```python
from build123d import *

# Parameters (mm, degrees)
SKIZZE1_W                       = 7.72
SKIZZE1_H                       = 10
SKIZZE1_W_2                     = 1.2
SKIZZE1_H_2                     = 20
SKIZZE1_W_3                     = 27.68
SKIZZE1_H_3                     = 5
AUFSATZ_LINEAR_AUSTRAGEN5_DEPTH = 3.2
SKIZZE2_W                       = 1.2
SKIZZE2_H                       = 20
AUFSATZ_LINEAR_AUSTRAGEN6_DEPTH = 10


with BuildPart() as part:
    # Skizze1 → Aufsatz-Linear austragen5 (new body)
    with BuildSketch(Plane(origin=(0, 0, 0), x_dir=(1, 0, 0), z_dir=(0, 1, 0))):
        with Locations((3.86, 15)):
            Rectangle(SKIZZE1_W, SKIZZE1_H)
        with Locations((-0.6, 10)):
            Rectangle(SKIZZE1_W_2, SKIZZE1_H_2)
        with Locations((3.86, 5)):
            Rectangle(SKIZZE1_W, SKIZZE1_H)
        Polygon((8.92, 20), (7.72, 20), (7.72, 10), (8.92, 10), (8.92, 15), align=None)
        Polygon((8.92, 10), (7.72, 10), (7.72, 0), (8.92, 0), (8.92, 5), align=None)
        with Locations((22.76, 12.5)):
            Rectangle(SKIZZE1_W_3, SKIZZE1_H_3)
        with Locations((22.76, 7.5)):
            Rectangle(SKIZZE1_W_3, SKIZZE1_H_3)
        Polygon((36.6, 20), (36.6, 15), (36.6, 10), (37.8, 10), (37.8, 20), align=None)
        Polygon((37.8, 10), (36.6, 10), (36.6, 5), (36.6, 0), (37.8, 0), align=None)
        with Locations((41.66, 15)):
            Rectangle(SKIZZE1_W, SKIZZE1_H)
        Polygon((45.52, 20), (45.52, 10), (46.72, 10), (46.72, 15), (46.72, 20), align=None)
        Polygon((46.72, 10), (45.52, 10), (45.52, 0), (46.72, 0), (46.72, 5), align=None)
        with Locations((41.66, 5)):
            Rectangle(SKIZZE1_W, SKIZZE1_H)
        with Locations((60.56, 12.5)):
            Rectangle(SKIZZE1_W_3, SKIZZE1_H_3)
        with Locations((60.56, 7.5)):
            Rectangle(SKIZZE1_W_3, SKIZZE1_H_3)
        with Locations((79.46, 15)):
            Rectangle(SKIZZE1_W, SKIZZE1_H)
        Polygon((74.4, 15), (74.4, 10), (75.6, 10), (75.6, 20), (74.4, 20), align=None)
        Polygon((75.6, 10), (74.4, 10), (74.4, 5), (74.4, 0), (75.6, 0), align=None)
        with Locations((79.46, 5)):
            Rectangle(SKIZZE1_W, SKIZZE1_H)
        Polygon((83.32, 20), (83.32, 10), (84.52, 10), (84.52, 15), (84.52, 20), align=None)
        Polygon((84.52, 10), (83.32, 10), (83.32, 0), (84.52, 0), (84.52, 5), align=None)
        with Locations((98.36, 12.5)):
            Rectangle(SKIZZE1_W_3, SKIZZE1_H_3)
        with Locations((98.36, 7.5)):
            Rectangle(SKIZZE1_W_3, SKIZZE1_H_3)
        with Locations((117.26, 15)):
            Rectangle(SKIZZE1_W, SKIZZE1_H)
        Polygon((112.2, 15), (112.2, 10), (113.4, 10), (113.4, 20), (112.2, 20), align=None)
        Polygon((113.4, 10), (112.2, 10), (112.2, 5), (112.2, 0), (113.4, 0), align=None)
        Polygon((121.12, 20), (121.12, 10), (122.32, 10), (122.32, 15), (122.32, 20), align=None)
        with Locations((117.26, 5)):
            Rectangle(SKIZZE1_W, SKIZZE1_H)
        Polygon((122.32, 10), (121.12, 10), (121.12, 0), (122.32, 0), (122.32, 5), align=None)
        with Locations((136.16, 12.5)):
            Rectangle(SKIZZE1_W_3, SKIZZE1_H_3)
        with Locations((136.16, 7.5)):
            Rectangle(SKIZZE1_W_3, SKIZZE1_H_3)
        Polygon((150, 15), (150, 10), (151.2, 10), (151.2, 20), (150, 20), align=None)
        Polygon((151.2, 10), (150, 10), (150, 5), (150, 0), (151.2, 0), align=None)
        with Locations((155.06, 15)):
            Rectangle(SKIZZE1_W, SKIZZE1_H)
        with Locations((159.52, 15)):
            Rectangle(SKIZZE1_W_2, SKIZZE1_H)
        with Locations((155.06, 5)):
            Rectangle(SKIZZE1_W, SKIZZE1_H)
        with Locations((159.52, 5)):
            Rectangle(SKIZZE1_W_2, SKIZZE1_H)
    extrude(amount=AUFSATZ_LINEAR_AUSTRAGEN5_DEPTH)

    # Skizze2 → Aufsatz-Linear austragen6 (add)
    with BuildSketch(Plane(origin=(0, 3.2, 0), x_dir=(1, 0, 0), z_dir=(0, 1, 0))):
        with Locations((8.32, 10)):
            Rectangle(SKIZZE2_W, SKIZZE2_H)
        with Locations((-0.6, 10)):
            Rectangle(SKIZZE2_W, SKIZZE2_H)
        with Locations((37.2, 10)):
            Rectangle(SKIZZE2_W, SKIZZE2_H)
        with Locations((46.12, 10)):
            Rectangle(SKIZZE2_W, SKIZZE2_H)
        with Locations((75, 10)):
            Rectangle(SKIZZE2_W, SKIZZE2_H)
        with Locations((83.92, 10)):
            Rectangle(SKIZZE2_W, SKIZZE2_H)
        with Locations((112.8, 10)):
            Rectangle(SKIZZE2_W, SKIZZE2_H)
        with Locations((121.72, 10)):
            Rectangle(SKIZZE2_W, SKIZZE2_H)
        with Locations((150.6, 10)):
            Rectangle(SKIZZE2_W, SKIZZE2_H)
        with Locations((159.52, 10)):
            Rectangle(SKIZZE2_W, SKIZZE2_H)
    extrude(amount=AUFSATZ_LINEAR_AUSTRAGEN6_DEPTH)


solid = part.part
```
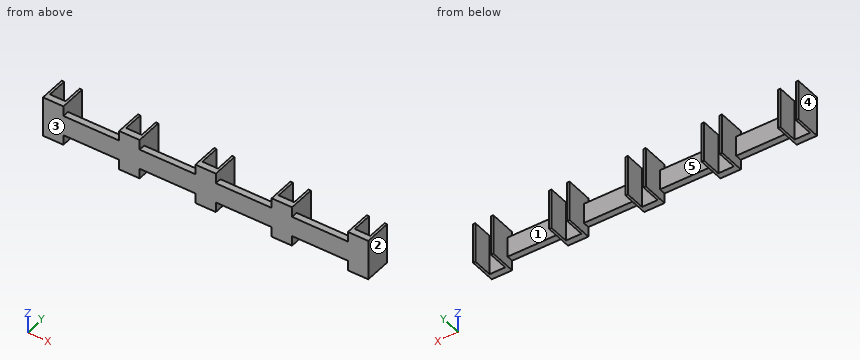
Read the model definition and answer for the solid it produces. Units are mm, in the model's axes. Face numbers are marked on the shaded views. A direction names the side the tool comes from. Round coordinates to 2 decimals unless told otherwise and drop trailing zeros. Loops run counter-clockwise (first coordinate to the right, second up) from the corner with the lowest first, then second, coordinate; pieces in that order, holes last. Notation, with made-up numbers: (5, 58) -> (33, 58) arc R34 ccw to (33, 91) -> close; hole circle Ø4 at (39, -27). An arc over 180 degrees is marked (long way). One line per item, written item: value.
1) Flat-ended cylindrical pins translate along their axes: P1, Ø4, axis at x = 4.5, z = -9, coming from the +Y side; P2, Ø5, axis at x = 110.5, z = -4.5, coming from the +Y side; P3, Ø2.5, axis at x = 29, y = 1.5, coming from the -Z side; P4, Ø1.6, axis at x = 138.5, y = 2, coming from the +Z side. Find the tip coordinate at first contact, or state that the pin passes through.
Answer list:
P1: stops at y = 3.2
P2: stops at y = 13.2
P3: stops at z = -15
P4: stops at z = -5
2) Consider L1, parallel to X at y = 1.25, z = -16.75; L2, parallel to Y at x = 131, z = -11.5. Determine where each line is inside the solid, lowest interval first. Write a range as [from, to].
Answer list:
L1: x = [-1.2, 8.92], [36.6, 46.72], [74.4, 84.52], [112.2, 122.32], [150, 160.12]
L2: y = [0, 3.2]
3) The mould has two halves that part along X. Classify the marked faces 1, 2 and 3: pulls with the +X half, pulls with the -X half, needs draft (parallel to the pull), parting line crosses it, or undercut.
Answer list:
face 1: undercut
face 2: pulls with the +X half
face 3: needs draft
4) A cutting plane is placed at A-A (y = 7). Give the number of separate pieces and of enclosed holes in the cut face, and give its area (3 significant figures).
Answer list:
separate pieces: 10
enclosed holes: 0
area: 240 mm²
5) For the marked faces 4 and 5, determine the directions among +Z, -Z, +X, -X, +Y, -Y from which every point of the face is accessible in a straight line to the end or side of a thin tool.
Answer list:
face 4: +Z, -Z, -X, +Y, -Y
face 5: +Z, -Z, +Y
6) A cutting plane is placed at C-C (x = 41). Determine the outline of the cut face in (y, z).
Answer list:
outline: (0, -20) -> (3.2, -20) -> (3.2, 0) -> (0, 0) -> close
